Verification items for this drawing (mm, ordinates from the low corner). A direction names the side the tool comes from. Round coordinates to 2 decimals unless told otherwise and drop trailing zeros. Loops run counter-clockwise (first coordinate to the right, second up) from the corner with the lowest first, then second, coordinate; pieces in that order, holes last. Notation, with made-up numbers: (18, 19.5) - (70, 19.5) arc R14 ccw to (70, 39.5) - close; hole circle Ø6 at (36.25, 82.5). An arc over 180 degrees is marked (long way). Put each result on its own line as item: value.
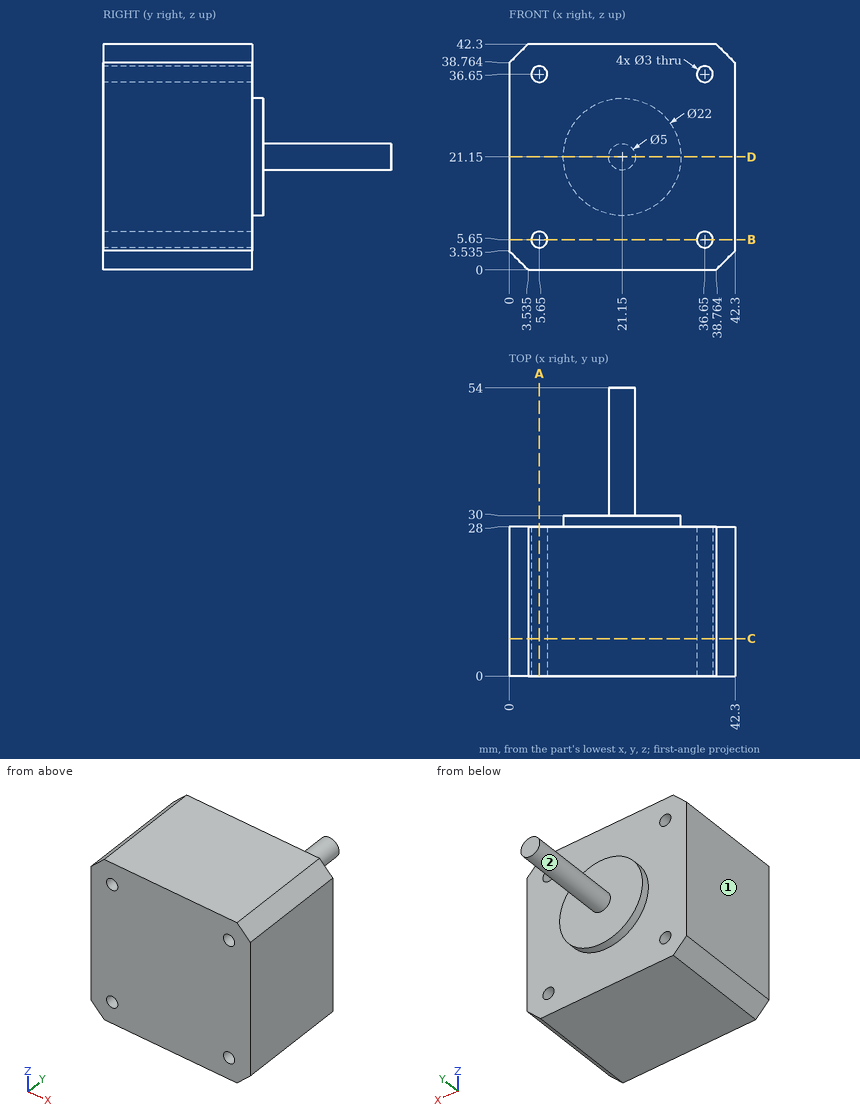
Item 1: Section check C-C on y = 7. Count the separate pieces of the cut face and the enclosed holes in it, then the cut area to 3 significant figures.
Filled sheet:
separate pieces: 1
enclosed holes: 4
area: 1,740 mm²
Item 2: Thickness scan on line 1 (Z direction, x = 36.65, y = 15.5); line 2 (X direction, y = 14, z = 36). Record the ranges inside material, lowest first. Write a range as from..to.
Filled sheet:
line 1: 0..4.15, 7.15..35.15, 38.15..42.3
line 2: 0..4.3, 7..35.3, 38..42.3
Item 3: Go/stop test with a flat-tipped pin: pin 1 (5 mm diameter, centred on x = 15.5, z = 14.5, fed in from +Y). Record where the tip stops, or that it passes through.
Filled sheet:
pin 1: y = 30
Item 4: Tool access check on the marked faces 1 and 2. Record the directions out of +Z, -Z, +X, -X, +Y, -Y that give a thin tool (end or side, any length) a straight path to the whole face; none if there is none.
Filled sheet:
face 1: +Z, -Z, -X, +Y, -Y
face 2: +Y
Item 5: Section check A-A on x = 5.65. Enter the section's corners in (y, z), then the cut area to 3 significant figures.
Filled sheet:
outline: (0, 0) - (28, 0) - (28, 4.15) - (0, 4.15) - close; (0, 7.15) - (28, 7.15) - (28, 35.15) - (0, 35.15) - close; (0, 38.15) - (28, 38.15) - (28, 42.3) - (0, 42.3) - close
area: 1,020 mm²
Item 6: Section check B-B on z = 5.65. Enter the section's corners in (x, y).
Filled sheet:
outline: (0, 0) - (4.15, 0) - (4.15, 28) - (0, 28) - close; (7.15, 0) - (35.15, 0) - (35.15, 28) - (7.15, 28) - close; (38.15, 0) - (42.3, 0) - (42.3, 28) - (38.15, 28) - close
Item 7: Section check D-D on z = 21.15. Enter the section's corners in (x, y).
Filled sheet:
outline: (0, 0) - (42.3, 0) - (42.3, 28) - (32.15, 28) - (32.15, 30) - (23.65, 30) - (23.65, 54) - (18.65, 54) - (18.65, 30) - (10.15, 30) - (10.15, 28) - (0, 28) - close
